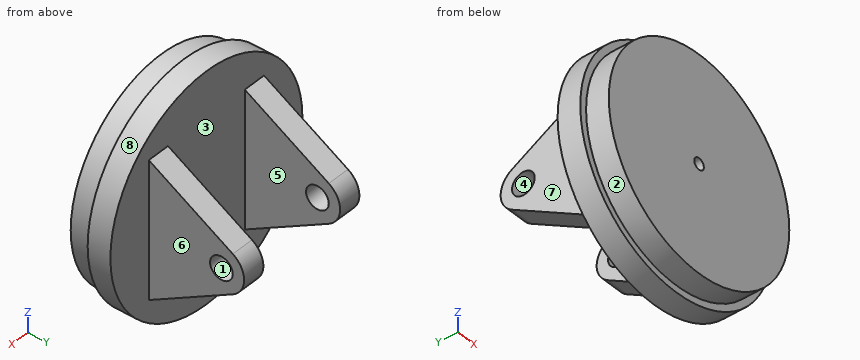
from build123d import *

# Parameters (mm, degrees)
SKETCH1_R           = 50
BOSS_EXTRUDE1_DEPTH = 10
BOSS_EXTRUDE2_START = 20
SKETCH2_R           = 5
BOSS_EXTRUDE2_DEPTH = 10
BOSS_EXTRUDE3_START = -20
SKETCH2_2_R         = 5
BOSS_EXTRUDE3_DEPTH = 10
SKETCH3_R           = 47
BOSS_EXTRUDE4_DEPTH = 10
SKETCH4_R           = 2.5
CUT_EXTRUDE1_DEPTH  = 10


with BuildPart() as part:
    # Sketch1 → Boss-Extrude1 (new body)
    with BuildSketch(Plane(origin=(0, 0, 0), x_dir=(1, 0, 0), z_dir=(0, 1, 0))):
        Circle(SKETCH1_R)
    extrude(amount=BOSS_EXTRUDE1_DEPTH)

    # Sketch2 → Boss-Extrude2 (add)
    with BuildSketch(Plane(origin=(0, 0, 0), x_dir=(0, 0, -1), z_dir=(1, 0, 0)).offset(BOSS_EXTRUDE2_START)):
        with BuildLine():
            Line((30, 10), (8.660254038, 46.961524227))
            ThreePointArc((8.660254038, 46.961524227), (0, 51.961524227), (-8.660254038, 46.961524227))
            Line((-8.660254038, 46.961524227), (-30, 10))
            Line((-30, 10), (30, 10))
        make_face()
        with Locations((0, 41.961524227)):
            Circle(SKETCH2_R, mode=Mode.SUBTRACT)
    extrude(amount=BOSS_EXTRUDE2_DEPTH)

    # Sketch2_2 → Boss-Extrude3 (add)
    with BuildSketch(Plane(origin=(0, 0, 0), x_dir=(0, 0, -1), z_dir=(1, 0, 0)).offset(BOSS_EXTRUDE3_START)):
        with BuildLine():
            Line((30, 10), (8.660254038, 46.961524227))
            ThreePointArc((8.660254038, 46.961524227), (0, 51.961524227), (-8.660254038, 46.961524227))
            Line((-8.660254038, 46.961524227), (-30, 10))
            Line((-30, 10), (30, 10))
        make_face()
        with Locations((0, 41.961524227)):
            Circle(SKETCH2_2_R, mode=Mode.SUBTRACT)
    extrude(amount=-BOSS_EXTRUDE3_DEPTH)

    # Sketch3 → Boss-Extrude4 (add)
    with BuildSketch(Plane.XZ):
        Circle(SKETCH3_R)
    extrude(amount=BOSS_EXTRUDE4_DEPTH)

    # Sketch4 → Cut-Extrude1 (cut)
    with BuildSketch(Plane.XZ.offset(10)):
        Circle(SKETCH4_R)
    extrude(amount=-CUT_EXTRUDE1_DEPTH, mode=Mode.SUBTRACT)


solid = part.part
Source: CAD feature listing. Evaluate the final solid. Frame: model axes, mm. Face numbers are marked on the shaded views. A direction names the side the tool comes from. Round coordinates to 2 decimals unless told otherwise and drop trailing zeros. Loops run counter-clockwise (first coordinate to the right, second up) from the corner with the lowest first, then second, coordinate; pieces in that order, holes last.
Q1. Access query for the marked faces 5, 6, 7 and 8. Directions: +Z, -Z, +X, -X, +Y, -Y. A direction counts if a zero-diameter tool reaches every point of the face in a straight line with its end or side. Return the directions, or none.
Q2. Mould query, pull axis Z, two halves, no side actions, for the marked faces 1, 2, 3 and 4. Classes: pulls with the +Z half, pulls with the -Z half, needs draft (parallel to the pull), parting line crosses it, or undercut.
Q3. First-contact query: P1, Ø4.5, axis at x = 0, z = 0, coming from the +Y side; P2, Ø11.5, axis at y = 41.96, z = 0, coming from the +X side; P3, Ø4, axis at x = 0, z = -1, coming from the -Y side; P4, Ø21, axis at y = 25.5, z = -13, coming from the -X side. Flat tips, straight axial feed; report the tip coordinate or a pass-through.
Q4. Ray query, line 1 (X direction, y = 39, z = 8.5); line 2 (Z direction, x = 0, y = -3); line 3 (Y direction, x = -34.5, z = -14). Return the intervals inside material, ascending.
Q5. Section D-D, the plane y = -2. Return loops of the section in (x, z), plus the area to 3 significant figures.
Q6. Section B-B, the plane y = 20. Return loops of the section in (x, z).
Q7. Section C-C, the plane x = -28. Return loops of the section in (y, z), plus the area to 3 significant figures.
Q8. Section A-A, the plane z = 0. Return loops of the section in (x, y).
Solutions:
1. face 5: +Z, -Z, +Y
1. face 6: +Z, -Z, +X, +Y
1. face 7: +Z, -Z, -X, +Y
1. face 8: +Y, -Y
2. face 1: undercut
2. face 2: parting line crosses it
2. face 3: needs draft
2. face 4: undercut
3. P1: stops at y = 10
3. P2: stops at x = 30
3. P3: stops at y = -10
3. P4: stops at x = -30
4. line 1: x = -30 to -20, 20 to 30
4. line 2: z = -47 to -2.5, 2.5 to 47
4. line 3: y = -10 to 10
5. outline: circle Ø94 at (0, 0); hole circle Ø5 at (0, 0)
5. area: 6,920 mm2
6. outline: (-30, -24.23) - (-20, -24.23) - (-20, 24.23) - (-30, 24.23) - close; (20, -24.23) - (30, -24.23) - (30, 24.23) - (20, 24.23) - close
7. outline: (-10, -37.75) - (0, -37.75) - (0, -41.42) - (10, -41.42) - (10, -30) - (46.96, -8.66) arc R10 ccw to (46.96, 8.66) - (10, 30) - (10, 41.42) - (0, 41.42) - (0, 37.75) - (-10, 37.75) - close; hole circle Ø10 at (41.96, 0)
7. area: 3,000 mm2
8. outline: (-50, 0) - (-47, 0) - (-47, -10) - (-2.5, -10) - (-2.5, 0) - (2.5, 0) - (2.5, -10) - (47, -10) - (47, 0) - (50, 0) - (50, 10) - (30, 10) - (30, 36.96) - (20, 36.96) - (20, 10) - (-20, 10) - (-20, 36.96) - (-30, 36.96) - (-30, 10) - (-50, 10) - close; (-30, 46.96) - (-20, 46.96) - (-20, 51.96) - (-30, 51.96) - close; (20, 46.96) - (30, 46.96) - (30, 51.96) - (20, 51.96) - close
